```python
from build123d import *

# Parameters (mm, degrees)
F0_W      = 12.7
F0_H      = 12.7
F1_DEPTH  = 38.1
F0_H_2    = 19.05
F2_DEPTH  = 38.1
F4_DEPTH  = 12.7
F6_DEPTH  = 12.7
F8_DEPTH  = 12.7
F10_DEPTH = 12.7


with BuildPart() as f1:
    # F0 (on Front) → F1 (new body)
    with BuildSketch(Plane.XZ):
        with Locations((-6.35, 6.35)):
            Rectangle(F0_W, F0_H)
    extrude(amount=F1_DEPTH)

    # F0 (on Front) → F2 (join)
    with BuildSketch(Plane.XZ):
        with Locations((6.35, 6.35)):
            Rectangle(F0_W, F0_H)
        with Locations((-6.35, 6.35)):
            Rectangle(F0_W, F0_H)
        with Locations((6.35, -9.525)):
            Rectangle(F0_W, F0_H_2)
        with Locations((19.05, 6.35)):
            Rectangle(F0_W, F0_H)
        with Locations((6.35, 22.225)):
            Rectangle(F0_W, F0_H_2)
    extrude(amount=F2_DEPTH)

    # F3 (on face) → F4 (cut)
    with BuildSketch(Plane.XY.offset(12.7)):
        Polygon((0, -38.1), (-12.7, -25.4), (-12.7, -38.1), align=None)
    extrude(amount=-F4_DEPTH, mode=Mode.SUBTRACT)

    # F5 (on face) → F6 (cut)
    with BuildSketch(Plane.XY.offset(12.7)):
        Polygon((25.4, -25.4), (12.7, -38.1), (25.4, -38.1), align=None)
    extrude(amount=-F6_DEPTH, mode=Mode.SUBTRACT)

    # F7 (on face) → F8 (cut)
    with BuildSketch(Plane(origin=(0, 0, 0), x_dir=(0, -1, 0), z_dir=(-1, 0, 0))):
        Polygon((38.1, 31.75), (25.4, 31.75), (38.1, 12.7), align=None)
    extrude(amount=-F8_DEPTH, mode=Mode.SUBTRACT)

    # F9 (on face) → F10 (cut)
    with BuildSketch(Plane(origin=(0, 0, 0), x_dir=(0, -1, 0), z_dir=(-1, 0, 0))):
        Polygon((38.1, -19.05), (38.1, 0), (25.4, -19.05), align=None)
    extrude(amount=-F10_DEPTH, mode=Mode.SUBTRACT)


solid = f1.part
```
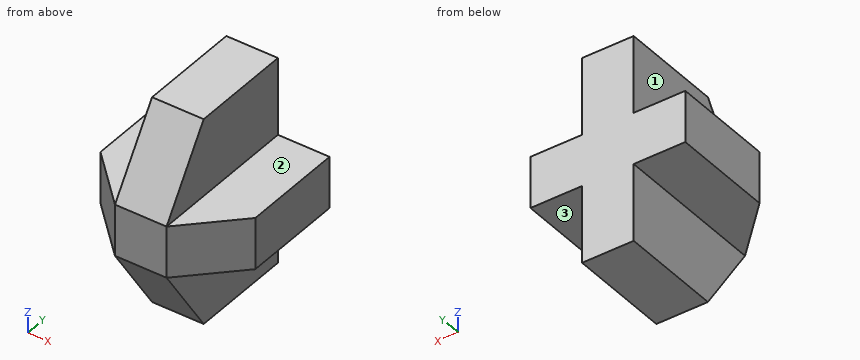
Design review of the part built by this model. Coordinates are the model's own, in mm. Face numbers are marked on the shaded views. A direction names the side the tool comes from. Round coordinates to 2 decimals unless told otherwise and drop trailing zeros. Write each loop counter-clockwise with the first axis right and the second up, starting at its lowest first coordinate (ties: lowest second). Pieces come first, ordered by that corner, then holes.
Item 1: We need section C-C on z = 22. Write out the cut boundary in (x, y), and give its area (3 significant figures).
Item 2: Clearance check with flat-ended pins moving along their axes: pin 1 Ø8 at (x, z) = (18, 25.5) entering from -Y; pin 2 Ø15 at (y, z) = (-13, 23) entering from -X; pin 3 Ø3 at (y, z) = (-27, 24) entering from +X; pin 4 Ø2 at (x, y) = (21, -16) entering from -Z. State where each tip first meets the part, or that it passes through.
Item 3: For the marked faces 1, 2 and 3, list the 3-axis set-ups (+Z, -Z, +X, -X, +Y, -Y) from which the entire face can be reached by the end or side of a thin tool; tool diameter is ignored.
Item 4: We need section D-D on x = -5. Write out the cut boundary in (y, z), and give its area (3 significant figures).
Item 5: For probe 1 along Z at (x, y) = (-1, -35); probe 2 along Y at (x, z) = (-7, 10), list the stretches that pass through material, from the lowest coordinate up.
Item 6: We need section B-B on x = 2. Write out the cut boundary in (y, z), and give its area (3 significant figures).
Item 7: We need section A-A on y = -14. Write out the cut boundary in (x, z).
Returned:
1. outline: (0, -31.9) - (12.7, -31.9) - (12.7, 0) - (0, 0) - close
1. area: 405 mm2
2. pin 1: passes through
2. pin 2: stops at x = 0
2. pin 3: stops at x = 12.7
2. pin 4: stops at z = 0
3. face 1: +Z, -X, +Y, -Y
3. face 2: +Z, +X, +Y, -Y
3. face 3: -Z, +X, +Y, -Y
4. outline: (-33.1, 0) - (0, 0) - (0, 12.7) - (-33.1, 12.7) - close
4. area: 420 mm2
5. probe 1: z = 0 to 12.7
5. probe 2: y = -31.1 to 0
6. outline: (-38.1, 0) - (-25.4, -19.05) - (0, -19.05) - (0, 31.75) - (-25.4, 31.75) - (-38.1, 12.7) - close
6. area: 1,690 mm2
7. outline: (-12.7, 0) - (0, 0) - (0, -19.05) - (12.7, -19.05) - (12.7, 0) - (25.4, 0) - (25.4, 12.7) - (12.7, 12.7) - (12.7, 31.75) - (0, 31.75) - (0, 12.7) - (-12.7, 12.7) - close
